```python
from build123d import *

# Parameters (mm, degrees)
SKETCH1_W                                           = 25.41
SKETCH1_H                                           = 18.5
BOSS_EXTRUDE1_DEPTH                                 = 12
F_2_56_TAPPED_HOLE1_D                               = 1.778
F_2_56_TAPPED_HOLE1_DEPTH                           = 7.46583491
F_2_56_TAPPED_HOLE1_TIP                             = 0.53416509
SKETCH5_R                                           = 3
CUT_EXTRUDE1_DEPTH                                  = 3
CBORE_FOR_2_BINDING_HEAD_MACHINE_SCREW2_D           = 2.4384
CBORE_FOR_2_BINDING_HEAD_MACHINE_SCREW2_CBORE_D     = 5.55752
CBORE_FOR_2_BINDING_HEAD_MACHINE_SCREW2_CBORE_DEPTH = 7.269988


with BuildPart() as part:
    # Sketch1 → Boss-Extrude1 (new body)
    with BuildSketch(Plane(origin=(0, 0, 0), x_dir=(1, 0, 0), z_dir=(0, 1, 0))):
        with Locations((12.705, 9.25)):
            Rectangle(SKETCH1_W, SKETCH1_H)
    extrude(amount=BOSS_EXTRUDE1_DEPTH)

    # #2-56 Tapped Hole1
    with Locations(Plane(origin=(0, 0, 0), x_dir=(-1, 0, 0), z_dir=(0, -1, 0))):
        with Locations((-23.91, 17), (-23.91, 1.5), (-1.5, 1.5), (-1.5, 17)):
            Hole(F_2_56_TAPPED_HOLE1_D / 2, depth=F_2_56_TAPPED_HOLE1_DEPTH)
            with Locations((0, 0, -(F_2_56_TAPPED_HOLE1_DEPTH + F_2_56_TAPPED_HOLE1_TIP / 2))):  # 118° drill point
                Cone(0, F_2_56_TAPPED_HOLE1_D / 2, F_2_56_TAPPED_HOLE1_TIP, mode=Mode.SUBTRACT)

    # Sketch5 → Cut-Extrude1 (cut)
    with BuildSketch(Plane.XZ):
        with Locations(Location((12.705, -9.25, 0), (0, 0, 270))):
            Circle(SKETCH5_R)
    extrude(amount=-CUT_EXTRUDE1_DEPTH, mode=Mode.SUBTRACT)

    # CBORE for #2 Binding Head Machine Screw2 (through all)
    with Locations(Plane(origin=(0, 0, 0), x_dir=(-1, 0, 0), z_dir=(0, -1, 0))):
        with Locations((-20.41, 9.25), (-5, 9.25)):
            CounterBoreHole(CBORE_FOR_2_BINDING_HEAD_MACHINE_SCREW2_D / 2, CBORE_FOR_2_BINDING_HEAD_MACHINE_SCREW2_CBORE_D / 2, CBORE_FOR_2_BINDING_HEAD_MACHINE_SCREW2_CBORE_DEPTH)


solid = part.part
```
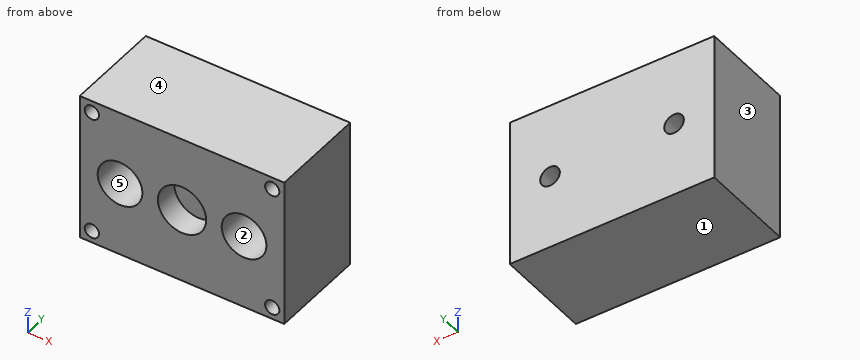
Geometry check sheet. Reference: the model listing, model coordinates, mm. Face numbers are marked on the shaded views. A direction names the side the tool comes from. Give positions to 0.01 mm unless a question says otherwise; leave off trailing zeros. Order: outer loops, then holes, each group sorted by start corner. A loop starts at its lowest first (then second) coordinate and runs counter-clockwise, first axis right, second up.
1. Section check C-C, the plane y = 4.25. Enter the section's corners in (x, z).
2. Gauge pin test, flat ends, axial feed: pin 1 Ø2.5 at (x, z) = (23.91, -17) entering from -Y; pin 2 Ø1.7 at (x, z) = (20, -10) entering from -Y; pin 3 Ø2 at (x, z) = (5, -9.25) entering from -Y; pin 4 Ø1.4 at (x, z) = (1.5, -1.5) entering from -Y. Record the tip position at first contact, or that the pin passes through.
3. Release check for a two-part mould opening along Z. For the marked faces 1, 2 and 3 record: pulls with the +Z half, pulls with the -Z half, needs draft (parallel to the pull), parting line crosses it, or undercut.
4. Thickness scan on L1, parallel to X at y = 0.8, z = -9.25 (3 decimals); L2, parallel to X at y = 4, z = -9.25; L3, parallel to X at y = 4.25, z = -11.75. Record the ranges inside material, lowest first.
5. Access from +Z, -Z, +X, -X, +Y, -Y to the whole of each face (thin tool, end or side, straight path). Record for the marked faces 4 and 5.
6. Section check D-D, the plane x = 13. Enter the section's corners in (y, z).
7. Section check B-B, the plane x = 5. Enter the section's corners in (y, z).
8. Section check A-A, the plane z = -9.25. Enter the section's corners in (x, y) (3 decimals), and give its area (3 significant figures).
Values follow:
1. outline: (0, -18.5) - (25.41, -18.5) - (25.41, 0) - (0, 0) - close; hole circle Ø1.78 at (1.5, -17); hole circle Ø1.78 at (1.5, -1.5); hole circle Ø5.56 at (5, -9.25); hole circle Ø5.56 at (20.41, -9.25); hole circle Ø1.78 at (23.91, -17); hole circle Ø1.78 at (23.91, -1.5)
2. pin 1: stops at y = 0
2. pin 2: stops at y = 7.27
2. pin 3: passes through
2. pin 4: stops at y = 7.58
3. face 1: pulls with the -Z half
3. face 2: undercut
3. face 3: needs draft
4. L1: x = 0 to 2.221, 7.779 to 9.705, 15.705 to 17.631, 23.189 to 25.41
4. L2: x = 0 to 2.22, 7.78 to 17.63, 23.19 to 25.41
4. L3: x = 0 to 3.79, 6.21 to 19.2, 21.62 to 25.41
5. face 4: +Z, +X, -X, +Y, -Y
5. face 5: -Y
6. outline: (0, -18.5) - (12, -18.5) - (12, 0) - (0, 0) - (0, -6.26) - (3, -6.26) - (3, -12.24) - (0, -12.24) - close
7. outline: (0, -18.5) - (12, -18.5) - (12, -10.47) - (7.27, -10.47) - (7.27, -12.03) - (0, -12.03) - close; (0, -6.47) - (7.27, -6.47) - (7.27, -8.03) - (12, -8.03) - (12, 0) - (0, 0) - close
8. outline: (0, 0) - (2.221, 0) - (2.221, 7.27) - (3.781, 7.27) - (3.781, 12) - (0, 12) - close; (6.219, 7.27) - (7.779, 7.27) - (7.779, 0) - (9.705, 0) - (9.705, 3) - (15.705, 3) - (15.705, 0) - (17.631, 0) - (17.631, 7.27) - (19.191, 7.27) - (19.191, 12) - (6.219, 12) - close; (21.629, 7.27) - (23.189, 7.27) - (23.189, 0) - (25.41, 0) - (25.41, 12) - (21.629, 12) - close
8. area: 183 mm2
